CAD build for the part. Positions are in the model's coordinates, mm. Face numbers are marked on the shaded views. Give positions to 0.01 mm unless a question says otherwise; leave off trailing zeros. Write each loop counter-clockwise with the first axis right and the second up, starting at its lowest first coordinate (ties: lowest second). Pieces come first, ordered by that corner, then holes. Notation, with made-up numbers: M 41.25,-35 L 64.25,-35 A5 ccw 64.25,-27 Z; hole C 4.5,-3.5 d8. An arc over 180 degrees is marked long. One line per question, with ' | ' between items. Start each with the question number.
1. Cut at D-D, the plane x = 0. Count the separate pieces of the cut face and the enclosed holes in it, then the cut area to 4 significant figures.
2. Flat gauge pins, fed straight in: pin 1 (4 mm diameter, centred on y = -8, z = 4, fed in from -X); pin 2 (5 mm diameter, centred on x = 8.63, y = 0, fed in from +Z); pin 3 (4 mm diameter, centred on y = -6.5, z = 5, fed in from -X). Where does each tip first touch, or does it go through?
3. Pull direction Y, two halves, no side cores. Call the marked faces 1, 2 and 3: released by +Y, released by -Y, zero draft, split by the parting line, or undercut.
4. Cut at B-B, the plane z = 4.5. Write the cut outline in (x, y), then the cut area to 3 significant figures.
5. Wall check: L1, parallel to Y at x = 0, z = 1.75; L2, parallel to Y at x = 10.5, z = 1. Give the ranges that are in metal, low to high.
6. Cut at A-A, the plane x = -9. Write the cut outline in (y, z), then the cut area to 3 significant figures.
7. Cut at C-C, the plane y = 15.5. Write the cut outline in (x, z), then the cut area to 3 significant figures.
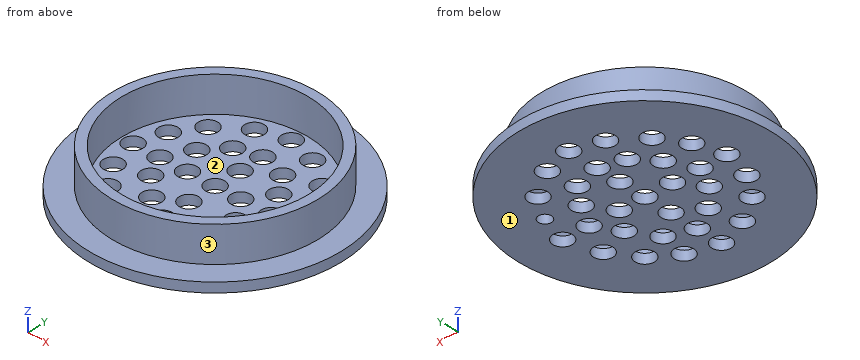
```python
from build123d import *

# Parameters (mm, degrees)
F0_R     = 19.5
F1_DEPTH = 1.5
F2_R     = 15.95
F2_R_2   = 14.5
F3_DEPTH = 7
F4_R     = 1.5
F4_R_2   = 1
F5_DEPTH = 25


with BuildPart() as f1:
    # F0 (on Top) → F1 (new body)
    with BuildSketch(Plane.XY):
        Circle(F0_R)
    extrude(amount=F1_DEPTH)

    # F2 (on Top) → F3 (join)
    with BuildSketch(Plane.XY):
        Circle(F2_R)
        Circle(F2_R_2, mode=Mode.SUBTRACT)
    extrude(amount=F3_DEPTH)

    # F4 (on Top) → F5 (cut)
    with BuildSketch(Plane.XY):
        Circle(F4_R)
        with Locations((0, 4.163333)):
            Circle(F4_R)
        with Locations((0, -4.35781)):
            Circle(F4_R)
        with Locations((0, -8.73511)):
            Circle(F4_R)
        with Locations((0, -12.762225)):
            Circle(F4_R)
        with Locations((0, 7.956992)):
            Circle(F4_R)
        with Locations((0, 12.684477)):
            Circle(F4_R)
        with Locations((-4.26875, 0)):
            Circle(F4_R)
        with Locations((-8.529321, 0)):
            Circle(F4_R)
        with Locations((-12.673165, 0)):
            Circle(F4_R)
        with Locations((3.960573, 0)):
            Circle(F4_R)
        with Locations((8.629692, 0)):
            Circle(F4_R)
        with Locations((12.715172, 0)):
            Circle(F4_R)
        with Locations((-6.486582, 3.929877)):
            Circle(F4_R)
        with Locations((-11.272429, 4.338425)):
            Circle(F4_R)
        with Locations((-8.704414, 8.190447)):
            Circle(F4_R)
        with Locations((-4.502206, 11.400468)):
            Circle(F4_R)
        with Locations((4.544213, 11.342104)):
            Circle(F4_R)
        with Locations((8.863147, 8.248813)):
            Circle(F4_R)
        with Locations((11.372799, 4.396788)):
            Circle(F4_R_2)
        with Locations((11.08098, -4.999814)):
            Circle(F4_R)
        with Locations((8.279508, -8.910201)):
            Circle(F4_R)
        with Locations((4.602577, -11.478217)):
            Circle(F4_R)
        with Locations((-4.735662, -11.128034)):
            Circle(F4_R)
        with Locations((-8.879505, -8.268198)):
            Circle(F4_R)
        with Locations((-11.447521, -4.64963)):
            Circle(F4_R)
        with Locations((-6.778402, -3.423986)):
            Circle(F4_R)
        with Locations((-3.68511, -6.575642)):
            Circle(F4_R)
        with Locations((3.960573, -7.27601)):
            Circle(F4_R)
        with Locations((6.411861, -3.48235)):
            Circle(F4_R)
        with Locations((6.470224, 3.638057)):
            Circle(F4_R)
        with Locations((4.135665, 6.789712)):
            Circle(F4_R)
        with Locations((-3.743474, 6.964805)):
            Circle(F4_R)
    extrude(amount=F5_DEPTH, mode=Mode.SUBTRACT)


solid = f1.part
```
Here are the results:
1) separate pieces: 8 | enclosed holes: 0 | area: 42.95 mm^2
2) pin 1: x = -14.78 | pin 2: z = 1.5 | pin 3: x = -15.3
3) face 1: zero draft | face 2: undercut | face 3: split by the parting line
4) outline: C 0,0 d31.9; hole C 0,0 d29 | area: 139 mm^2
5) L1: -15.95 to -14.5, 14.5 to 15.95 | L2: -16.43 to -6.38, -3.62 to 3.91, 4.88 to 16.43
6) outline: M -17.3,0 L -9.76,0 L -9.76,1.5 L -11.37,1.5 L -11.37,7 L -13.17,7 L -13.17,1.5 L -17.3,1.5 Z; M -6.77,0 L -1.42,0 L -1.42,1.5 L -6.77,1.5 Z; M 1.42,0 L 6.72,0 L 6.72,1.5 L 1.42,1.5 Z; M 9.66,0 L 17.3,0 L 17.3,1.5 L 13.17,1.5 L 13.17,7 L 11.37,7 L 11.37,1.5 L 9.66,1.5 Z | area: 58.5 mm^2
7) outline: M -11.83,0 L 11.83,0 L 11.83,1.5 L 3.76,1.5 L 3.76,7 L -3.76,7 L -3.76,1.5 L -11.83,1.5 Z | area: 76.9 mm^2
